The drawing under review shows one solid part. Ordinate dimensions are in mm from its lowest x, y, z. A direction names the side the tool comes from. Give positions to 0.01 mm unless a question says otherwise; leave off trailing zeros. Write each loop counter-clockwise with the first axis right and the second up, starting at its lowest first coordinate (ties: lowest second). Pieces come first, ordered by that corner, then holes. Notation, with made-up numbers: (-34.5, 63) -> (14.5, 63) arc R22 ccw to (14.5, 85) -> close; hole circle Ø6 at (-20.5, -3). An arc over 180 degrees is marked (long way). Use CSV: the item, a comma, the result in double quotes.
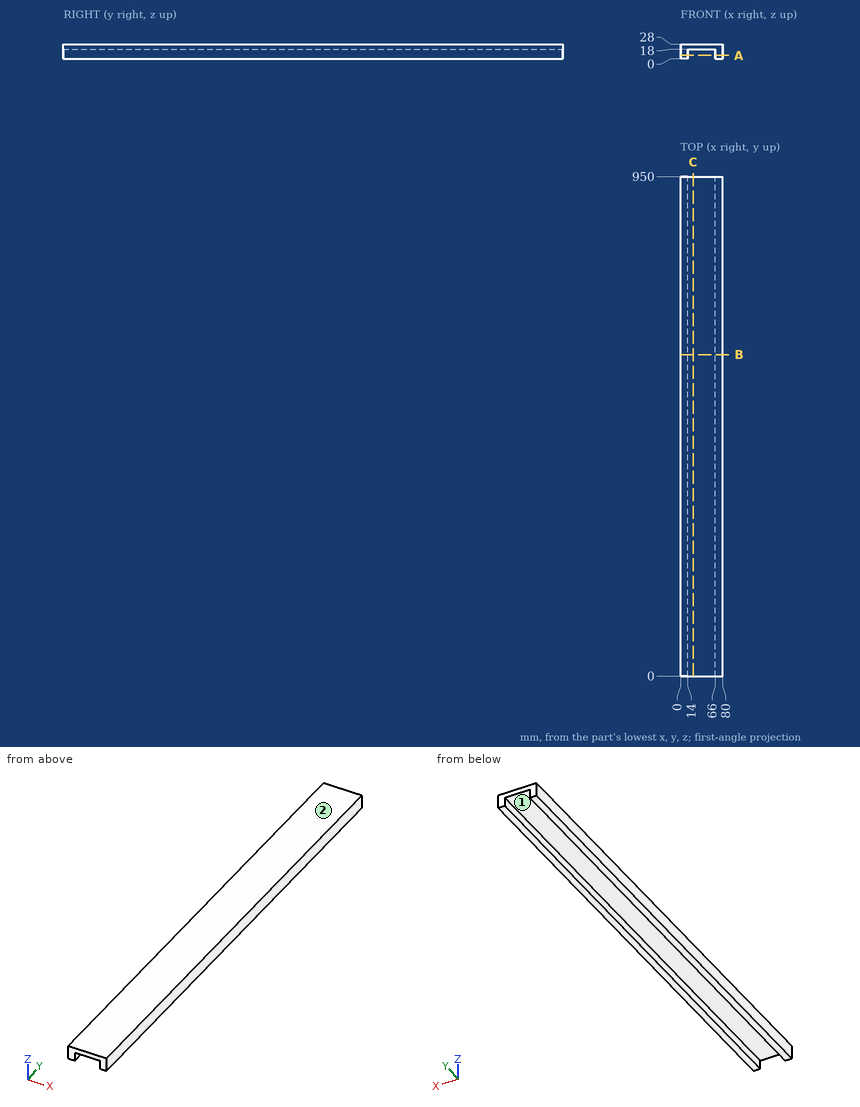
(1) For line 1 along X through (y, z) = (264, 5.25); line 2 along Z through (x, y) = (24.5, 315), list the stretches that pass through material, from the lowest coordinate up. Write a range as [from, to].
Established:
line 1,"x = [0, 14], [66, 80]"
line 2,"z = [18, 28]"
(2) Take a section at C-C (x = 24). Write out the cut boundary in (y, z).
Established:
outline,"(0, 18) -> (950, 18) -> (950, 28) -> (0, 28) -> close"
(3) Tool access review of the marked faces 1 and 2: name each direction out of +Z, -Z, +X, -X, +Y, -Y from which nothing blocks a thin tool from reaching the whole face with its end or side.
Established:
face 1,"-Z, +Y, -Y"
face 2,"+Z, +X, -X, +Y, -Y"
(4) Clearance check with a flat-ended pin moving along its axis: pin 1 (8 mm diameter, centred on x = 34.5, y = 365.5, fed in from -Z). State where the tip first meets the part, or that it passes through.
Established:
pin 1,"stops at z = 18"
(5) Take a section at B-B (y = 611.5). Write out the cut boundary in (x, z).
Established:
outline,"(0, 0) -> (14, 0) -> (14, 18) -> (66, 18) -> (66, 0) -> (80, 0) -> (80, 28) -> (0, 28) -> close"
(6) Take a section at A-A (z = 6.5). Write out the cut boundary in (x, y), then the cut area to 3 significant figures.
Established:
outline,"(0, 0) -> (14, 0) -> (14, 950) -> (0, 950) -> close; (66, 0) -> (80, 0) -> (80, 950) -> (66, 950) -> close"
area,"26,600 mm2"
